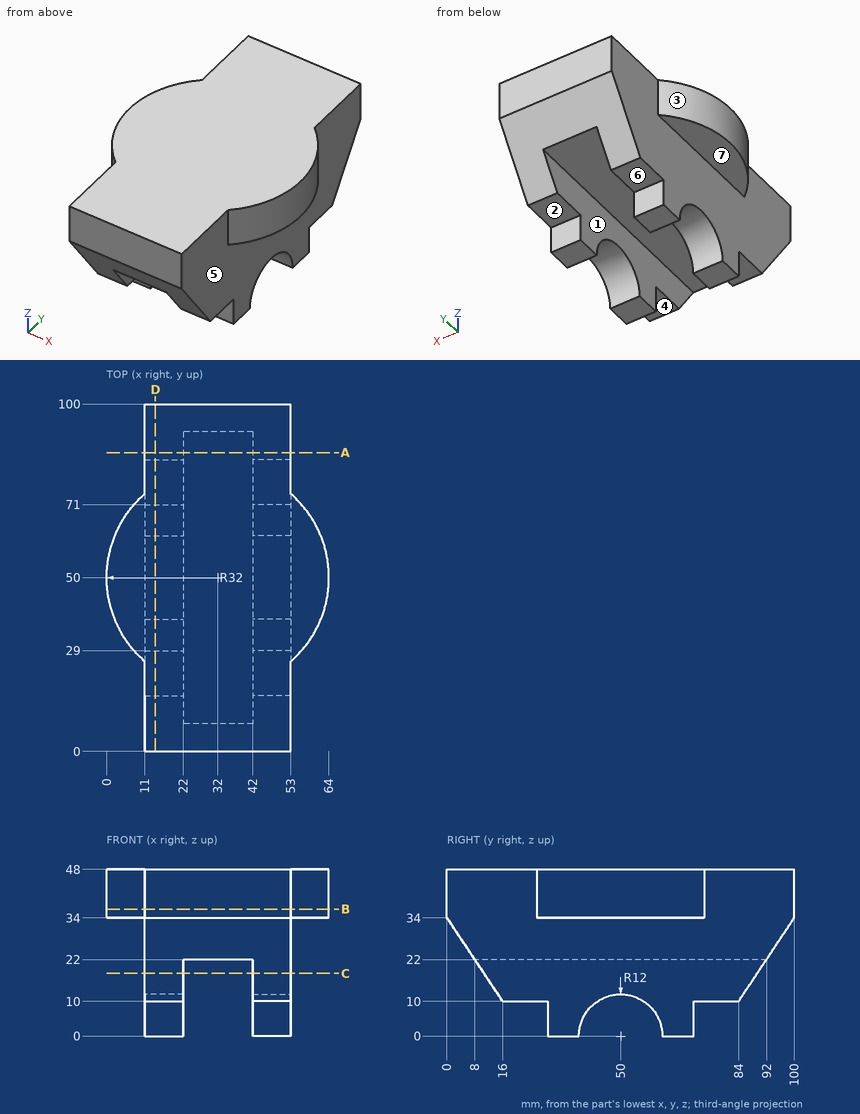
Design review of the part shown in the three views and the two pictorial views. Dimensions are in mm from the part's minimum x, y and z. A direction names the side the tool comes from. Give positions to 0.01 mm unless a question says otherwise; leave off trailing zeros. Loops run counter-clockwise (first coordinate to the right, second up) from the corner with the lowest first, then second, coordinate; pieces in that order, holes last. Notation, with made-up numbers: M -15.75,38.5 L 33.25,38.5 A21 cw 33.25,47.5 Z; hole C -6.75,-34 d4. An arc over 180 degrees is marked long. Write item = value, one per line.
Q1. Draft analysis for pull direction X (two halves, no side actions). For the marked faces 1, 2 and 3, state which applies: +X half, -X half, draft (parallel to the pull), parting line (faces both ways), or undercut.
Output values:
face_1 = undercut
face_2 = draft
face_3 = -X half
Q2. We need section D-D (x = 14). Give the boundary of the cut face in (y, z).
Output values:
outline = M 0,34 L 16,10 L 29,10 L 29,0 L 38,0 A12 cw 62,0 L 71,0 L 71,10 L 84,10 L 100,34 L 100,48 L 0,48 Z
Q3. We need section B-B (z = 36.5). Give the boundary of the cut face in (x, y), plus the area to 3 significant figures.
Output values:
outline = M 11,0 L 53,0 L 53,25.85 A32 ccw 53,74.15 L 53,100 L 11,100 L 11,74.15 A32 ccw 11,25.85 Z
area = 4,940 mm^2
Q4. For the marked faces 4, 5, 6 and 7, list the 3-axis set-ups (+Z, -Z, +X, -X, +Y, -Y) from which the entire face can be reached by the end or side of a thin tool; tool diameter is ignored.
Output values:
face_4 = -Z, +X, -X, -Y
face_5 = -Z, +X
face_6 = -Z, +X, -X, +Y
face_7 = -Z, -X, +Y, -Y
Q5. Insertion check: pin 1 (14.5 mm diameter, centred on y = 49, z = 35.5, fed in from -X); pin 2 (9 mm diameter, centred on x = 47.5, y = 78.5, fed in from -Z); pin 3 (10 mm diameter, centred on y = 24.5, z = 28.5, fed in from -X). Each pin has a flat end and moves straight along its axis. Give the tip position at first contact, or say it passes through.
Output values:
pin_1 = 0
pin_2 = 10
pin_3 = 11
Q6. We need section A-A (y = 86). Give the boundary of the cut face in (x, z).
Output values:
outline = M 11,13 L 22,13 L 22,22 L 42,22 L 42,13 L 53,13 L 53,48 L 11,48 Z
Q7. We need section C-C (z = 18). Give the boundary of the cut face in (x, y).
Output values:
outline = M 11,10.67 L 22,10.67 L 22,89.33 L 11,89.33 Z; M 42,10.67 L 53,10.67 L 53,89.33 L 42,89.33 Z
Q8. To check wall thickness, follow line 1 (X direction, y = 48, z = 16); line 2 (X direction, y = 86, z = 38); line 3 (Z direction, x = 6.5, y = 42). State the ranges of each line that lie inside material, in increasing order. Write a range as [from, to].
Output values:
line_1 = [11, 22], [42, 53]
line_2 = [11, 53]
line_3 = [34, 48]
